from build123d import *

# Parameters (mm, degrees)
SKETCH1_R           = 37
BOSS_EXTRUDE1_DEPTH = 3
BOSS_EXTRUDE2_DEPTH = 6.5
SKETCH3_R           = 4
SKETCH3_R_2         = 2
CUT_EXTRUDE1_DEPTH  = 6.5


with BuildPart() as part:
    # Sketch1 → Boss-Extrude1 (new body)
    with BuildSketch(Plane(origin=(0, 0, 0), x_dir=(1, 0, 0), z_dir=(0, 1, 0))):
        with Locations(Location((0, 0, 0), (0, 0, 270))):
            Circle(SKETCH1_R)
    extrude(amount=BOSS_EXTRUDE1_DEPTH)

    # Sketch1_3 → Boss-Extrude2 (add)
    with BuildSketch(Plane(origin=(0, 0, 0), x_dir=(1, 0, 0), z_dir=(0, 1, 0))):
        with BuildLine():
            ThreePointArc((24.729789728, 1), (0, 24.75), (-24.729789728, 1))
            Line((-24.729789728, 1), (-23.728938029, 1))
            ThreePointArc((-23.728938029, 1), (0, 23.75), (23.728938029, 1))
            Line((23.728938029, 1), (24.729789728, 1))
        make_face()
        with BuildLine():
            Line((-23.728938029, -1), (-24.729789728, -1))
            ThreePointArc((-24.729789728, -1), (0, -24.75), (24.729789728, -1))
            Line((24.729789728, -1), (23.728938029, -1))
            ThreePointArc((23.728938029, -1), (0, -23.75), (-23.728938029, -1))
        make_face()
        with BuildLine():
            ThreePointArc((-24.729789728, 1), (-24.75, 0), (-24.729789728, -1))
            Line((-24.729789728, -1), (-23.728938029, -1))
            ThreePointArc((-23.728938029, -1), (-23.75, 0), (-23.728938029, 1))
            Line((-23.728938029, 1), (-24.729789728, 1))
        make_face()
        with BuildLine():
            Line((23.728938029, -1), (24.729789728, -1))
            ThreePointArc((24.729789728, -1), (24.744946916, -0.500102103), (24.75, 0))
            ThreePointArc((24.75, 0), (24.744946916, 0.500102103), (24.729789728, 1))
            Line((24.729789728, 1), (23.728938029, 1))
            ThreePointArc((23.728938029, 1), (23.744733924, 0.500110889), (23.75, 0))
            ThreePointArc((23.75, 0), (23.744733924, -0.500110889), (23.728938029, -1))
        make_face()
        with BuildLine():
            ThreePointArc((-23.728938029, 1), (-23.75, 0), (-23.728938029, -1))
            Line((-23.728938029, -1), (-13.964240044, -1))
            ThreePointArc((-13.964240044, -1), (-14, 0), (-13.964240044, 1))
            Line((-13.964240044, 1), (-23.728938029, 1))
        make_face()
        with BuildLine():
            Line((13.964240044, -1), (23.728938029, -1))
            ThreePointArc((23.728938029, -1), (23.744733924, -0.500110889), (23.75, 0))
            ThreePointArc((23.75, 0), (23.744733924, 0.500110889), (23.728938029, 1))
            Line((23.728938029, 1), (13.964240044, 1))
            ThreePointArc((13.964240044, 1), (13.991057155, 0.500319591), (14, 0))
            ThreePointArc((14, 0), (13.991057155, -0.500319591), (13.964240044, -1))
        make_face()
    extrude(amount=BOSS_EXTRUDE2_DEPTH)

    # Sketch3 → Cut-Extrude1 (cut)
    with BuildSketch(Plane(origin=(0, 3, 0), x_dir=(1, 0, 0), z_dir=(0, 1, 0))):
        with Locations(Location((0, 0, 0), (0, 0, 270))):
            Circle(SKETCH3_R)
        with Locations(Location((8, 0, 0), (0, 0, 270))):
            Circle(SKETCH3_R_2)
        with Locations(Location((0, -8, 0), (0, 0, 270))):
            Circle(SKETCH3_R_2)
        with Locations(Location((-8, 0, 0), (0, 0, 270))):
            Circle(SKETCH3_R_2)
        with Locations(Location((0, 8, 0), (0, 0, 270))):
            Circle(SKETCH3_R_2)
    extrude(amount=-CUT_EXTRUDE1_DEPTH, mode=Mode.SUBTRACT)


solid = part.part
Source: CAD feature listing. Evaluate the final solid. Frame: model axes, mm. A direction names the side the tool comes from. Coordinates: 2 decimals unless noted, no trailing zeros. Loops run counter-clockwise (first coordinate to the right, second up) from the corner with the lowest first, then second, coordinate; pieces in that order, holes last. Notation, with made-up numbers: (-35.75, -9.5) - (10.25, -9.5) arc R13 cw to (10.25, 6.5) - close; hole circle Ø6 at (26.25, -36). An arc over 180 degrees is marked (long way). One line per item, written item: value. Start each with the question number.
1. Section D-D (z = 8). Return the cut outline in (x, y).
2. Ray query, L1, parallel to X at y = 1.65, z = 0; L2, parallel to Y at x = 19.5, z = 6; L3, parallel to X at y = 3.5, z = 5. Return the intervals inside material, ascending.
3. Section B-B (x = 0). Return the cut outline in (y, z), and give its area (3 significant figures).
4. Section C-C (x = -8). Return the cut outline in (y, z).
5. Section A-A (y = 4.75). Return the cut outline in (x, z), and give its area (3 significant figures).
6. Mould query, pull axis Z, two halves, no side actions, for faces 3 (the flat face through (15, 6.5, 0)), 4 (the cylindrical face through (-14.17, 1.48, 34.18)), 5 (the cylindrical face through (0.508, 4.726, 23.745)). Classes: pulls with the +Z half, pulls with the -Z half, needs draft (parallel to the pull), parting line crosses it, or undercut.
7. Contact query for flat-ended pins moving along their axis: P1, Ø1, axis at x = -21.5, y = 5.5, coming from the -Z side; P2, Ø14, axis at x = 2.5, z = -3.5, coming from the +Y side; P3, Ø1.8, axis at x = 17.5, y = 4.5, coming from the +Z side. Output: stop coordinate, or through.
8. Set-up query: faces 1 (the flat face through (19, 5, -1)), 2 (the cylindrical face through (-3.905, 1.521, -0.867)). Return all of +Z, -Z, +X, -X, +Y, -Y with unobstructed straight access to the full face (end or side cutting, diameter ignored); none if empty.
Verdict:
1. outline: (-36.12, 0) - (-2, 0) - (-2, 3) - (-22.36, 3) - (-22.36, 6.5) - (-23.42, 6.5) - (-23.42, 3) - (-36.12, 3) - close; (2, 0) - (36.12, 0) - (36.12, 3) - (23.42, 3) - (23.42, 6.5) - (22.36, 6.5) - (22.36, 3) - (2, 3) - close
2. L1: x = -37 to -10, -6 to -4, 4 to 6, 10 to 37
2. L2: y = 0 to 3
2. L3: x = -24.24 to -23.22, 23.22 to 24.24
3. outline: (0, -37) - (3, -37) - (3, -24.75) - (6.5, -24.75) - (6.5, -23.75) - (3, -23.75) - (3, -10) - (0, -10) - close; (0, -6) - (3, -6) - (3, -4) - (0, -4) - close; (0, 4) - (3, 4) - (3, 6) - (0, 6) - close; (0, 10) - (3, 10) - (3, 23.75) - (6.5, 23.75) - (6.5, 24.75) - (3, 24.75) - (3, 37) - (0, 37) - close
3. area: 181 mm2
4. outline: (0, -36.12) - (3, -36.12) - (3, -23.42) - (6.5, -23.42) - (6.5, -22.36) - (3, -22.36) - (3, -2) - (0, -2) - close; (0, 2) - (3, 2) - (3, 22.36) - (6.5, 22.36) - (6.5, 23.42) - (3, 23.42) - (3, 36.12) - (0, 36.12) - close
5. outline: circle Ø49.5 at (0, 0); hole (-23.73, -1) arc R23.75 ccw to (23.73, -1) - (13.96, -1) arc R14 ccw to (13.96, 1) - (23.73, 1) arc R23.75 ccw to (-23.73, 1) - (-13.96, 1) arc R14 ccw to (-13.96, -1) - close
5. area: 191 mm2
6. face 3: needs draft
6. face 4: parting line crosses it
6. face 5: undercut
7. P1: stops at z = -13.1
7. P2: stops at y = 3
7. P3: stops at z = 18.36
8. face 1: +Y
8. face 2: +Y, -Y
